Can you work these out from the model? Positions are in its coordinate system, mm. A direction names the side the tool comes from. Coordinates: 2 decimals unless noted, no trailing zeros. Order: outer loops, then holes, each group sorted by start corner. A loop starts at its lowest first (then second) coordinate and runs counter-clockwise, first axis right, second up. Notation, with made-up numbers: (65.25, 43.5) -> (69.25, 43.5) arc R16 ccw to (69.25, 69.5) -> close; hole circle Ø2 at (59, 45). An arc over 180 degrees is marked (long way). Write item = value, one per line.
```python
from build123d import *

# Parameters (mm, degrees)
FILLET2_R  = 1.8
SKETCH2_W  = 12
SKETCH2_H  = 1.6
SLOT_DEPTH = 1.4


with BuildPart() as part:
    # BodySke → Base-Revolve (revolve)
    with BuildSketch(Plane.XY, mode=Mode.PRIVATE) as base_revolve_sk:
        Polygon((3.6, 3), (3.6, 6), (0, 5.685040811), (0, 0), (13.6, 0), (13.6, 3), align=None)
    revolve(base_revolve_sk.sketch.rotate(Axis((-25.4, 0, 0), (1, 0, 0)), 90), axis=Axis((-25.4, 0, 0), (1, 0, 0)))  # turned: the seam where the file's is

    # Fillet2
    fillet2_edges = [part.edges().sort_by_distance(p)[0] for p in [
        (0, 0, -5.685040811),
    ]]
    fillet(fillet2_edges, radius=FILLET2_R)

    # Sketch2 → Slot (cut)
    with BuildSketch(Plane(origin=(0, 0, 0), x_dir=(0, 0, -1), z_dir=(1, 0, 0))):
        Rectangle(SKETCH2_W, SKETCH2_H)
    extrude(amount=SLOT_DEPTH, mode=Mode.SUBTRACT)


solid = part.part
```
Item 1: For faces 4 (the flat face through (13.6, 0, 0)), 5 (the flat face through (1, -0.8, 0)), 6 (the cylindrical face through (8.53, -0.9, 2.86)), which set-ups out of +Z, -Z, +X, -X, +Y, -Y let a thin tool reach every point of the face, with its end or its side?
A:
face_4 = +Z, -Z, +X, +Y, -Y
face_5 = +Z, -Z, -X
face_6 = +X
Item 2: I want a section at A-A, the plane y = 0. Please give me the cut outline in (x, z).
A:
outline = (1.4, -5.79) arc R1.8 ccw to (1.64, -5.83) -> (3.6, -6) -> (3.6, -3) -> (13.6, -3) -> (13.6, 3) -> (3.6, 3) -> (3.6, 6) -> (1.64, 5.83) arc R1.8 ccw to (1.4, 5.79) -> close
Item 3: I'm going to push flat-ended pins straight in: P1, Ø0.7, axis at x = 1, z = 3, coming from the +Y side; P2, Ø1.5, axis at x = 3.5, z = 4, coming from the +Y side; P3, Ø1, axis at x = 8.5, y = 1.5, coming from the -Z side. Where does each tip first touch, or does it pass through?
A:
P1 = 5.05
P2 = 5.04
P3 = -2.83
Item 4: I want a section at C-C, the plane x = 7.25. Please give me the cut outline in (y, z), plus the area to 3 significant figures.
A:
outline = circle Ø6 at (0, 0)
area = 28.3 mm2
Item 5: If I drill on probe 1 along Y at (x, z) = (12.75, 0); probe 2 along X at (y, z) = (0, -1.5); probe 3 along X at (y, z) = (4, 0.75), over which ranges is the centre line in solid material (lowest first)?
A:
probe_1 = -3 to 3
probe_2 = 1.4 to 13.6
probe_3 = 0 to 3.6
Item 6: I want a section at D-D, the plane x = 2.75. Please give me the cut outline in (y, z), plus the area to 3 significant figures.
A:
outline = circle Ø11.85 at (0, 0)
area = 110 mm2
Item 7: I want a section at B-B, the plane z = 0. Please give me the cut outline in (x, y), plus the area to 3 significant figures.
A:
outline = (0, -4.04) arc R1.8 ccw to (1.64, -5.83) -> (3.6, -6) -> (3.6, -3) -> (13.6, -3) -> (13.6, 3) -> (3.6, 3) -> (3.6, 6) -> (1.64, 5.83) arc R1.8 ccw to (0, 4.04) -> (0, 0.8) -> (1.4, 0.8) -> (1.4, -0.8) -> (0, -0.8) -> close
area = 98.7 mm2
Item 8: If we mould it in two halves opening along Y, with no side actions, what happens to faces 1 (the flat face through (1, 0.8, 0)), 2 (the flat face through (3.6, -3, -1)), 3 (the conical face through (2.173, -5.825, -0.765))? For each: pulls with the +Y half, pulls with the -Y half, needs draft (parallel to the pull), parting line crosses it, or undercut.
A:
face_1 = undercut
face_2 = needs draft
face_3 = parting line crosses it
